```python
from build123d import *

# Parameters (mm, degrees)
SKETCH1_R           = 1.6
SKETCH1_R_2         = 1.8
SKETCH1_R_3         = 6.35
BOSS_EXTRUDE1_DEPTH = 6


with BuildPart() as part:
    # Sketch1 → Boss-Extrude1 (new body)
    with BuildSketch(Plane.XY):
        Polygon((0, -44.45), (22.2, -44.45), (22.2, -23.85), (63.5, -23.85), (63.5, -44.45), (167.8, -44.45), (177.8, -34.45), (177.8, 34.45), (167.8, 44.45), (63.5, 44.45), (63.5, 23.85), (22.2, 23.85), (22.2, 44.45), (0, 44.45), align=None)
        with Locations((18.85, 29.15)):
            Circle(SKETCH1_R, mode=Mode.SUBTRACT)
        with Locations((18.85, 39.15)):
            Circle(SKETCH1_R, mode=Mode.SUBTRACT)
        with Locations((66.85, 29.15)):
            Circle(SKETCH1_R, mode=Mode.SUBTRACT)
        with Locations((66.85, 39.15)):
            Circle(SKETCH1_R, mode=Mode.SUBTRACT)
        with Locations((153.3, 34.15)):
            Circle(SKETCH1_R_2, mode=Mode.SUBTRACT)
        with Locations((109, 25.4)):
            Circle(SKETCH1_R, mode=Mode.SUBTRACT)
        with Locations((18.85, -29.15)):
            Circle(SKETCH1_R, mode=Mode.SUBTRACT)
        with Locations((18.85, -39.15)):
            Circle(SKETCH1_R, mode=Mode.SUBTRACT)
        with Locations((66.85, -29.15)):
            Circle(SKETCH1_R, mode=Mode.SUBTRACT)
        with Locations((66.85, -39.15)):
            Circle(SKETCH1_R, mode=Mode.SUBTRACT)
        with Locations((153.3, -34.15)):
            Circle(SKETCH1_R_2, mode=Mode.SUBTRACT)
        with Locations((109, -25.4)):
            Circle(SKETCH1_R, mode=Mode.SUBTRACT)
        with Locations((86, -12)):
            Circle(SKETCH1_R, mode=Mode.SUBTRACT)
        with Locations((86, 32)):
            Circle(SKETCH1_R, mode=Mode.SUBTRACT)
        with Locations((80, 0)):
            Circle(SKETCH1_R_3, mode=Mode.SUBTRACT)
        with Locations((130, 0)):
            Circle(SKETCH1_R_3, mode=Mode.SUBTRACT)
    extrude(amount=BOSS_EXTRUDE1_DEPTH)


solid = part.part
```
The model under review builds one solid part; all positions refer to its coordinate system, in mm. A direction names the side the tool comes from. Round coordinates to 2 decimals unless told otherwise and drop trailing zeros. Write each loop counter-clockwise with the first axis right and the second up, starting at its lowest first coordinate (ties: lowest second). Pieces come first, ordered by that corner, then holes. Notation, with made-up numbers: M 83.25,-15.5 L 95.25,-15.5 A7 ccw 95.25,-2.5 Z; hole C 6.25,33.5 d2. An arc over 180 degrees is marked long. Use CSV: the item, a comma, the result in double quotes. Start each with the question number.
(1) We need section C-C, the plane x = 130. State the section outline as (y, z) points.
(2) For line 1 along Y through (x, z) = (66.85, 3.7); line 2 along Y through (x, z) = (109, 1.55); line 3 along Y through (x, z) = (80, 3.5), list the stretches that pass through material, from the lowest coordinate up.
(3) We need section D-D, the plane z = 2.75. State how many separate pieces and enclosed holes the cut face has, then the cut area to 3 significant figures.
(4) The part is to be moulded in two halves that separate along X. For faces 4 (the face through (0, 1, 3)), 5 (the face through (88, 1, 6)), 6 (the face through (177.8, 0, 3)), 7 (the face through (63.5, -34, 3)), say which applies: +X half, -X half, draft (parallel to the pull), parting line (faces both ways), or undercut.
(5) We need section A-A, the plane x = 18.85. State the section outline as (y, z) points.
(6) Tool access review of faces 1 (the face through (68.376, -28.669, 2.958)), 2 (the face through (22.2, -34, 3)), 3 (the face through (43, 23.85, 3)): name each direction out of +Z, -Z, +X, -X, +Y, -Y from which nothing blocks a thin tool from reaching the whole face with its end or side.
(7) We need section B-B, the plane y = 0. State the section outline as (x, z) points.
(8) Clearance check with flat-ended pins moving along their axes: P1, Ø1.8, axis at x = 48, z = 2, coming from the -Y side; P2, Ø1.8, axis at y = 39, z = 1.5, coming from the +X side. State where each tip first meets the part, or that it passes through.
Findings:
1,outline,"M -44.45,0 L -6.35,0 L -6.35,6 L -44.45,6 Z; M 6.35,0 L 44.45,0 L 44.45,6 L 6.35,6 Z"
2,line 1,"-44.45 to -40.75, -37.55 to -30.75, -27.55 to 27.55, 30.75 to 37.55, 40.75 to 44.45"
2,line 2,"-44.45 to -27, -23.8 to 23.8, 27 to 44.45"
2,line 3,"-44.45 to -6.35, 6.35 to 44.45"
3,separate pieces,"1"
3,enclosed holes,"16"
3,area,"13,600 mm^2"
4,face 4,"-X half"
4,face 5,"draft"
4,face 6,"+X half"
4,face 7,"undercut"
5,outline,"M -44.45,0 L -40.75,0 L -40.75,6 L -44.45,6 Z; M -37.55,0 L -30.75,0 L -30.75,6 L -37.55,6 Z; M -27.55,0 L 27.55,0 L 27.55,6 L -27.55,6 Z; M 30.75,0 L 37.55,0 L 37.55,6 L 30.75,6 Z; M 40.75,0 L 44.45,0 L 44.45,6 L 40.75,6 Z"
6,face 1,"+Z, -Z"
6,face 2,"+Z, -Z, -Y"
6,face 3,"+Z, -Z, +Y"
7,outline,"M 0,0 L 73.65,0 L 73.65,6 L 0,6 Z; M 86.35,0 L 123.65,0 L 123.65,6 L 86.35,6 Z; M 136.35,0 L 177.8,0 L 177.8,6 L 136.35,6 Z"
8,P1,"y = -23.85"
8,P2,"x = 174.15"
